The listing builds one solid part. Answer for the finished solid, in the listing's coordinates (mm). A direction names the side the tool comes from. Give positions to 0.01 mm unless a question says otherwise; leave off trailing zeros. Order: outer loops, then holes, each group sorted by start corner. A loop starts at its lowest first (then second) coordinate and runs counter-clockwise, first axis right, second up. Notation, with made-up numbers: (-14, 58) - (41, 58) arc R19 ccw to (41, 83) - close; hole circle Ø3 at (62, 29.25). An arc over 180 degrees is marked (long way). Use a Markdown table: item, result. Add a question column.
1) Straight lines are drawn through the part: line 1 (Y direction, x = 0, z = 0.6); line 2 (Y direction, x = -1.5, z = 0.6); line 3 (X direction, y = -0.25, z = 0.5). For each, find the intervals that lie inside material, in ascending order.
2) Find section A-A, the plane x = 1.5. Determine the outline of the cut face in (y, z).
3) Find section D-D, the plane y = -4.5. Determine the outline of the cut face in (x, z), plus the area to 3 significant figures.
4) Find section C-C, the plane x = -1. Determine the outline of the cut face in (y, z), plus the area to 3 significant figures.
5) For faces 5 (the face through (14.3, -6.369, 0.4)), 6 (the face through (9.7, -5.556, 0.4)), 7 (the face through (11.112, 9.7, 0.4)), 8 (the face through (-5.077, 2.258, 0.401)), 9 (the face through (6, 1, 0.813)), determine the directions among +Z, -Z, +X, -X, +Y, -Y from which every point of the face is accessible in a straight line to the end or side of a thin tool.
6) The mould has two halves that part along X. Classify faces 1 (the face through (3.8, 5.556, 0.4)), 2 (the face through (17.462, 3.9, 0.4)), 3 (the face through (12.7, 0.1, 0.4)), 4 (the face through (-0.232, -7.357, 0.401)): released by +X, released by -X, zero draft, split by the parting line, or undercut.
7) Find section B-B, the plane z = 0.3. State how many separate pieces and enclosed holes the cut face has, plus the area to 3 significant figures.
from build123d import *

# Parameters (mm, degrees)
SKETCH1_R           = 1.5875
SKETCH1_R_2         = 1.7859375
BOSS_EXTRUDE1_DEPTH = 0.8128
FILLET1_R           = 0.4064
FILLET2_R           = 3.571875


with BuildPart() as part:
    # Sketch1 → Boss-Extrude1 (new body)
    with BuildSketch(Plane.XY):
        with BuildLine():
            ThreePointArc((17.462464722, 10.31875), (14.287464722, 13.49375), (11.112464722, 10.31875))
            Line((11.112464722, 10.31875), (11.112464722, 5.55625))
            Line((11.112464722, 5.55625), (0, 5.55625))
            ThreePointArc((0, 5.55625), (-5.113201992, 2.17418478), (-4.001636336, -3.854714088))
            ThreePointArc((-4.001636336, -3.854714088), (-3.061446663, -5.6851033), (-3.287058398, -7.730434724))
            ThreePointArc((-3.287058398, -7.730434724), (-0.713207299, -12.628071623), (3.571875, -9.128125))
            ThreePointArc((3.571875, -9.128125), (4.61805296, -6.602427972), (7.143749984, -5.55625))
            Line((7.143749984, -5.55625), (12.699964722, -5.55625))
            Line((12.699964722, -5.55625), (12.699964722, -6.36905))
            Line((12.699964722, -6.36905), (15.874964722, -6.36905))
            Line((15.874964722, -6.36905), (15.874964722, -5.130880657))
            ThreePointArc((15.874964722, -5.130880657), (17.037095379, -3.96875), (17.462464722, -2.38125))
            Line((17.462464722, -2.38125), (17.462464722, 10.31875))
        make_face()
        with Locations((14.287464722, 0.03175)):
            Circle(SKETCH1_R, mode=Mode.SUBTRACT)
        with Locations((14.287464722, 7.90575)):
            Circle(SKETCH1_R, mode=Mode.SUBTRACT)
        Circle(SKETCH1_R_2, mode=Mode.SUBTRACT)
        with Locations((0, -9.128125)):
            Circle(SKETCH1_R_2, mode=Mode.SUBTRACT)
    extrude(amount=BOSS_EXTRUDE1_DEPTH)

    # Fillet1
    fillet1_edges = [part.edges().sort_by_distance(p)[0] for p in [
        (15.874964722, -5.130880657, 0.4064),
        (15.874964722, -6.36905, 0.4064),
        (12.699964722, -5.55625, 0.4064),
        (12.699964722, -6.36905, 0.4064),
    ]]
    fillet(fillet1_edges, radius=FILLET1_R - 0.0001)  # a hair under: the kernel refuses the full size

    # Fillet2
    fillet2_edges = [part.edges().sort_by_distance(p)[0] for p in [
        (11.112464722, 5.55625, 0.4064),
    ]]
    fillet(fillet2_edges, radius=FILLET2_R)


solid = part.part
The answers:
| question | item | result |
|---|---|---|
| 1 | line 1 | -12.7 to -10.91, -7.34 to -1.79, 1.79 to 5.56 |
| 1 | line 2 | -12.37 to -10.1, -8.16 to -0.97, 0.97 to 5.35 |
| 1 | line 3 | -5.55 to -1.77, 1.77 to 12.73, 15.85 to 17.46 |
| 2 | outline | (-12.37, 0) - (-10.1, 0) - (-10.1, 0.81) - (-12.37, 0.81) - close; (-8.16, 0) - (-0.97, 0) - (-0.97, 0.81) - (-8.16, 0.81) - close; (0.97, 0) - (5.56, 0) - (5.56, 0.81) - (0.97, 0.81) - close |
| 3 | outline | (-3.51, 0) - (16.65, 0) - (16.65, 0.81) - (-3.51, 0.81) - close |
| 3 | area | 16.4 mm2 |
| 4 | outline | (-12.56, 0) - (-10.61, 0) - (-10.61, 0.81) - (-12.56, 0.81) - close; (-7.65, 0) - (-1.48, 0) - (-1.48, 0.81) - (-7.65, 0.81) - close; (1.48, 0) - (5.47, 0) - (5.47, 0.81) - (1.48, 0.81) - close |
| 4 | area | 9.84 mm2 |
| 5 | face 5 | +Z, -Z, +X, -Y |
| 5 | face 6 | +Z, -Z, -Y |
| 5 | face 7 | +Z, -Z, -X, +Y |
| 5 | face 8 | +Z, -Z, -X |
| 5 | face 9 | +Z, +X, -X, +Y, -Y |
| 6 | face 1 | zero draft |
| 6 | face 2 | released by +X |
| 6 | face 3 | undercut |
| 6 | face 4 | undercut |
| 7 | separate pieces | 1 |
| 7 | enclosed holes | 4 |
| 7 | area | 304 mm2 |
